Work out the finished part from the listing and answer in its coordinate system (mm). Coordinates: 2 decimals unless noted, no trailing zeros. Order: outer loops, then holes, each group sorted by start corner. A loop starts at its lowest first (then second) coordinate and runs counter-clockwise, first axis right, second up. Notation, with made-up numbers: (26.5, 73) -> (37.5, 73) arc R20 cw to (37.5, 105) -> close; hole circle Ø10 at (41.5, 26). An arc over 180 degrees is marked (long way). Write item = value, one per line. Start each with the question number.
Q1. Flat-ended cylindrical pins translate along their axes: pin 1 (0.8 mm diameter, centred on x = 56.5, z = 1, fed in from -Y); pin 2 (0.8 mm diameter, centred on y = -62.5, z = 0.5, fed in from +X); pin 3 (0.8 mm diameter, centred on x = -30, z = 1, fed in from -Y). Find the tip coordinate at first contact, or state that the pin passes through.
Q2. Straight lines are drawn through the part: L1, parallel to Y at x = 12.7, z = 0.7; L2, parallel to X at y = 11, z = 1.05; L3, parallel to X at y = 18, z = 0.45. For each, find the intervals that lie inside material, in ascending order. Write a range as from..to.
Q3. The part is cut by section B-B, the plane y = 22. Determine the outline of the cut face in (x, z).
Q4. The part is cut by section A-A, the plane x = 28. Determine the outline of the cut face in (y, z).
Q5. The part is cut by section C-C, the plane z = 0.8. Determine the outline of the cut face in (x, y) (3 decimals).
Q6. The part is cut by section D-D, the plane y = -81. Determine the outline of the cut face in (x, z).
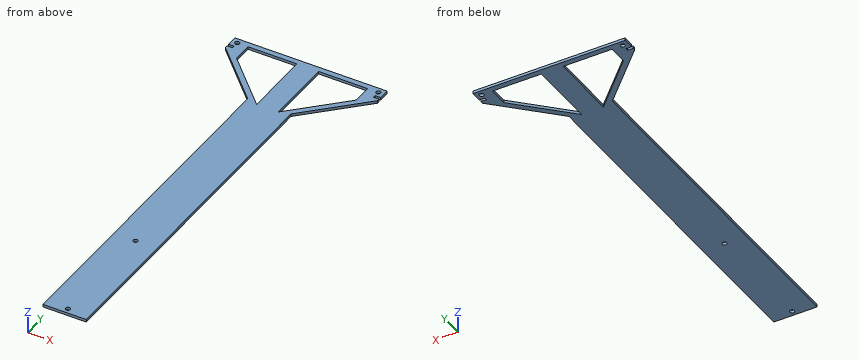
```python
from build123d import *

# Parameters (mm, degrees)
F0_R     = 1.35255
F1_DEPTH = 1.5875
F2_W     = 3.175
F2_H     = 1.5875
F3_DEPTH = 1.5875


with BuildPart() as f1:
    # F0 (on Top) → F1 (new body)
    with BuildSketch(Plane.XY):
        Polygon((0, 0), (0, -203.2), (25.4, -203.2), (25.4, 0), (57.21985, 31.81985), (57.21985, 41.34485), (-31.81985, 41.34485), (-31.81985, 31.81985), align=None)
        with Locations((12.7, -200.025)):
            Circle(F0_R, mode=Mode.SUBTRACT)
        with Locations((12.7, -132.8928)):
            Circle(F0_R, mode=Mode.SUBTRACT)
        with Locations((-28.64485, 38.16985)):
            Circle(F0_R, mode=Mode.SUBTRACT)
        with Locations((54.04485, 38.16985)):
            Circle(F0_R, mode=Mode.SUBTRACT)
    extrude(amount=F1_DEPTH)

    # F2 (on face) → F3 (cut, through all)
    with BuildSketch(Plane.XY.offset(1.5875)):
        with Locations((-30.23235, 34.2011)):
            Rectangle(F2_W, F2_H)
        with Locations((55.63235, 34.2011)):
            Rectangle(F2_W, F2_H)
        Polygon((-22.29485, 38.16985), (-22.29485, 26.784978), (6.35, -1.859872), (6.35, 38.16985), align=None)
        Polygon((47.69485, 38.16985), (19.05, 38.16985), (19.05, -1.859872), (47.69485, 26.784978), align=None)
    extrude(amount=-F3_DEPTH, mode=Mode.SUBTRACT)


solid = f1.part
```
Model answer:
q1.pin_1 = 30.7
q1.pin_2 = 25.4
q1.pin_3 = 29.6
q2.L1 = -203.2..-201.38, -198.67..-134.25, -131.54..41.34
q2.L2 = -11..-6.51, 6.35..19.05, 31.91..36.4
q2.L3 = -18..-13.51, 6.35..19.05, 38.91..43.4
q3.outline = (-22, 0) -> (-17.51, 0) -> (-17.51, 1.59) -> (-22, 1.59) -> close; (6.35, 0) -> (19.05, 0) -> (19.05, 1.59) -> (6.35, 1.59) -> close; (42.91, 0) -> (47.4, 0) -> (47.4, 1.59) -> (42.91, 1.59) -> close
q4.outline = (2.6, 0) -> (7.09, 0) -> (7.09, 1.59) -> (2.6, 1.59) -> close; (38.17, 0) -> (41.34, 0) -> (41.34, 1.59) -> (38.17, 1.59) -> close
q5.outline = (-31.82, 31.82) -> (0, 0) -> (0, -203.2) -> (25.4, -203.2) -> (25.4, 0) -> (57.22, 31.82) -> (57.22, 33.407) -> (54.045, 33.407) -> (54.045, 34.995) -> (57.22, 34.995) -> (57.22, 41.345) -> (-31.82, 41.345) -> (-31.82, 34.995) -> (-28.645, 34.995) -> (-28.645, 33.407) -> (-31.82, 33.407) -> close; hole circle Ø2.705 at (-28.645, 38.17); hole (-22.295, 26.785) -> (6.35, -1.86) -> (6.35, 38.17) -> (-22.295, 38.17) -> close; hole circle Ø2.705 at (12.7, -200.025); hole circle Ø2.705 at (12.7, -132.893); hole (19.05, -1.86) -> (47.695, 26.785) -> (47.695, 38.17) -> (19.05, 38.17) -> close; hole circle Ø2.705 at (54.045, 38.17)
q6.outline = (0, 0) -> (25.4, 0) -> (25.4, 1.59) -> (0, 1.59) -> close
